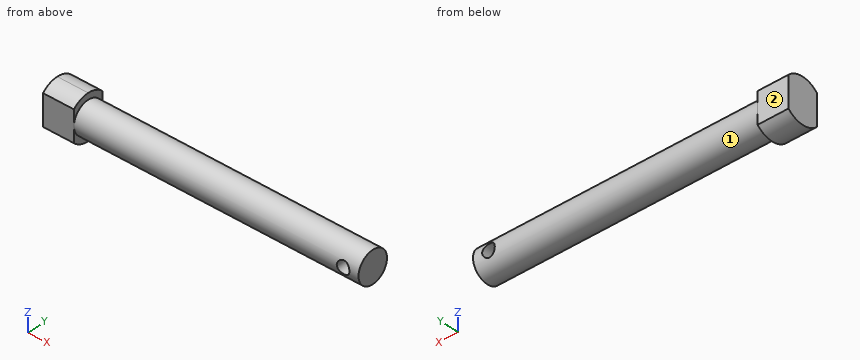
from build123d import *

# Parameters (mm, degrees)
SKETCH2_R               = 2.5
BOSS_EXTRUDE1_DEPTH     = 25
BOSS_EXTRUDE4_START     = -4.9
BOSS_EXTRUDE4_DEPTH     = 4.9
CUT_EXTRUDE2_DEPTH      = 26.734218465
CUT_EXTRUDE2_DEPTH_BACK = 26.734218465
SKETCH5_R               = 1


with BuildPart() as part:
    # Sketch2 → Boss-Extrude1 (new, symmetric)
    with BuildSketch(Plane(origin=(0, 0, 0), x_dir=(0, 0, -1), z_dir=(1, 0, 0))):
        Circle(SKETCH2_R)
    extrude(amount=BOSS_EXTRUDE1_DEPTH, both=True)

    # Sketch3 → Boss-Extrude4 (add)
    with BuildSketch(Plane.ZY.offset(25).offset(BOSS_EXTRUDE4_START)):
        with BuildLine():
            Line((0, 2.5), (-2.449489743, 2.5))
            ThreePointArc((-2.449489743, 2.5), (-3.5, 0), (-2.449489743, -2.5))
            Line((-2.449489743, -2.5), (0, -2.5))
            ThreePointArc((0, -2.5), (-2.5, 0), (0, 2.5))
        make_face()
        with BuildLine():
            Line((2.449489743, 2.5), (0, 2.5))
            ThreePointArc((0, 2.5), (1.767766953, 1.767766953), (2.5, 0))
            ThreePointArc((2.5, 0), (1.767766953, -1.767766953), (0, -2.5))
            Line((0, -2.5), (2.449489743, -2.5))
            ThreePointArc((2.449489743, -2.5), (3.226702194, -1.355873501), (3.5, 0))
            ThreePointArc((3.5, 0), (3.226702194, 1.355873501), (2.449489743, 2.5))
        make_face()
    extrude(amount=BOSS_EXTRUDE4_DEPTH)

    # Sketch5 → Cut-Extrude2 (cut, two sides: drawn at the far end of the back side and taken through both)
    with BuildSketch(Plane(origin=(0, 2.5, 0), x_dir=(1, 0, 0), z_dir=(0, 1, 0)).offset(-CUT_EXTRUDE2_DEPTH_BACK)):
        with Locations(Location((22.55, 0, 0), (0, 0, 180.000000001))):
            Circle(SKETCH5_R)
    extrude(amount=CUT_EXTRUDE2_DEPTH + CUT_EXTRUDE2_DEPTH_BACK, mode=Mode.SUBTRACT)


solid = part.part
Geometry check sheet. Reference: the model listing, model coordinates, mm. Face numbers are marked on the shaded views. A direction names the side the tool comes from. Coordinates: 2 decimals unless noted, no trailing zeros. Order: outer loops, then holes, each group sorted by start corner. A loop starts at its lowest first (then second) coordinate and runs counter-clockwise, first axis right, second up. Notation, with made-up numbers: (89, -28) -> (138, -28) arc R22 ccw to (138, 2) -> close; hole circle Ø7 at (-27, 76.25). An arc over 180 degrees is marked (long way). Use a Markdown table: item, result. Add a question column.
1. Go/stop test with flat-tipped pins: pin 1 Ø1.5 at (x, y) = (-5.5, 0.5) entering from +Z; pin 2 Ø3 at (x, z) = (8.5, -2.5) entering from -Y; pin 3 Ø1.1 at (y, z) = (1, -2.5) entering from +X; pin 4 Ø1 at (x, z) = (12.5, 2.5) entering from +Y. Record where each tip stops, or that it passes through.
2. Cross-section at C-C (x = -0.5). Enter the section's corners in (y, z), and give its area (3 significant figures).
3. Cross-section at D-D (z = -3). Enter the section's corners in (x, y), and give its area (3 significant figures).
4. Material ranges on L1, parallel to Z at x = 22.55, y = -0.05; L2, parallel to Z at x = 0, y = 0.45; L3, parallel to Z at x = 22.55, y = 1.3, recorded low to high.
5. Cross-section at A-A (y = -1.2). Enter the section's corners in (x, z).
6. Set-up check for the marked faces 1 and 2: record each of +Z, -Z, +X, -X, +Y, -Y from which the full face is reachable in a straight line by a thin tool's end or side.
7. Cross-section at B-B (y = 1.65). Enter the section's corners in (x, z).
Filled sheet:
| question | item | result |
|---|---|---|
| 1 | pin 1 | z = 2.5 |
| 1 | pin 2 | y = -2.29 |
| 1 | pin 3 | x = 25 |
| 1 | pin 4 | y = 1.5 |
| 2 | outline | circle Ø5 at (0, 0) |
| 2 | area | 19.6 mm2 |
| 3 | outline | (-25, -1.8) -> (-20.1, -1.8) -> (-20.1, 1.8) -> (-25, 1.8) -> close |
| 3 | area | 17.7 mm2 |
| 4 | L1 | -2.5 to -1, 1 to 2.5 |
| 4 | L2 | -2.46 to 2.46 |
| 4 | L3 | -2.14 to -1, 1 to 2.14 |
| 5 | outline | (-25, -3.29) -> (-20.1, -3.29) -> (-20.1, -2.19) -> (25, -2.19) -> (25, 2.19) -> (-20.1, 2.19) -> (-20.1, 3.29) -> (-25, 3.29) -> close; hole circle Ø2 at (22.55, 0) |
| 6 | face 1 | +X |
| 6 | face 2 | +Z, -Z, +X, -X, +Y |
| 7 | outline | (-25, -3.09) -> (-20.1, -3.09) -> (-20.1, -1.88) -> (25, -1.88) -> (25, 1.88) -> (-20.1, 1.88) -> (-20.1, 3.09) -> (-25, 3.09) -> close; hole circle Ø2 at (22.55, 0) |
